from build123d import *

# Parameters (mm, degrees)
SKETCH_1_R               = 120
EXTRUDE_1_DEPTH          = 20
CUT_EXTRUDE_1_DEPTH      = 171.880074906
CUT_EXTRUDE_1_DEPTH_BACK = 171.880074906
SKETCH_2_R               = 15
CUT_EXTRUDE_2_DEPTH      = 15
PATTERN_CIRCULAR_1_COUNT = 3
SKETCH_5_R               = 1.5
CUT_EXTRUDE_3_DEPTH      = 171.880074906
PATTERN_CIRCULAR_2_COUNT = 3
CUT_EXTRUDE_4_DEPTH      = 171.880074906
PATTERN_CIRCULAR_3_COUNT = 3
SKETCH_7_R               = 20
CUT_EXTRUDE_5_DEPTH      = 171.880074906
SKETCH_8_R               = 1.5
CUT_EXTRUDE_6_DEPTH      = 171.880074906
PATTERN_CIRCULAR_4_COUNT = 3
SKETCH_12_W              = 5
SKETCH_12_H              = 25
EXTRUDE_3_DEPTH          = 10
EXTRUDE_4_DEPTH          = 4
PATTERN_CIRCULAR_5_COUNT = 3


with BuildPart() as part:
    # Sketch 1 → Extrude 1 (new body)
    with BuildSketch(Plane(origin=(0, 0, 0), x_dir=(1, 0, 0), z_dir=(0, 1, 0))):
        with Locations(Location((0, 0, 0), (0, 0, 270))):
            Circle(SKETCH_1_R)
    extrude(amount=EXTRUDE_1_DEPTH)

    # Sketch 2 → Cut-Extrude 1 (cut, two sides: drawn at the far end of the back side and taken through both)
    with BuildSketch(Plane(origin=(0, 20, 0), x_dir=(1, 0, 0), z_dir=(0, 1, 0)).offset(-CUT_EXTRUDE_1_DEPTH_BACK)):
        with Locations(Location((60, 0, 0), (0, 0, 270))):
            Circle(SKETCH_2_R)
        with Locations(Location((-30, -51.961524227, 0), (0, 0, 270))):
            Circle(SKETCH_2_R)
        with Locations(Location((-30, 51.961524227, 0), (0, 0, 270))):
            Circle(SKETCH_2_R)
    extrude(amount=CUT_EXTRUDE_1_DEPTH + CUT_EXTRUDE_1_DEPTH_BACK, mode=Mode.SUBTRACT)

    # Sketch 4 → Cut-Extrude 2 (cut)
    with BuildSketch(Plane.XZ):
        Polygon((7.009618943, 42.141016151), (32.990381057, 27.141016151), (82.990381057, 113.74355653), (57.009618943, 128.74355653), align=None)
    cut_extrude_2 = extrude(amount=-CUT_EXTRUDE_2_DEPTH, mode=Mode.SUBTRACT)

    # Pattern Circular 1: Cut-Extrude 2 ×3 about axis
    pattern_circular_1_axis = Axis((0, 0, 0), (0, 1, 0))
    for i in range(1, PATTERN_CIRCULAR_1_COUNT):
        add(cut_extrude_2.rotate(pattern_circular_1_axis, i * 360 / PATTERN_CIRCULAR_1_COUNT), mode=Mode.SUBTRACT)

    # Sketch 5 → Cut-Extrude 3 (cut, symmetric)
    with BuildSketch(Plane.XZ):
        with Locations(Location((-45, 0, 0), (0, 0, 270))):
            Circle(SKETCH_5_R)
        with Locations(Location((-75, 0, 0), (0, 0, 270))):
            Circle(SKETCH_5_R)
        with Locations(Location((-105, 0, 0), (0, 0, 270))):
            Circle(SKETCH_5_R)
    cut_extrude_3 = extrude(amount=CUT_EXTRUDE_3_DEPTH, both=True, mode=Mode.SUBTRACT)

    # Pattern Circular 2: Cut-Extrude 3 ×3 about axis
    pattern_circular_2_axis = Axis((0, 0, 0), (0, 1, 0))
    for i in range(1, PATTERN_CIRCULAR_2_COUNT):
        add(cut_extrude_3.rotate(pattern_circular_2_axis, i * 360 / PATTERN_CIRCULAR_2_COUNT), mode=Mode.SUBTRACT)

    # Sketch 6 → Cut-Extrude 4 (cut, symmetric)
    with BuildSketch(Plane(origin=(0, 20, 0), x_dir=(1, 0, 0), z_dir=(0, 1, 0))):
        with BuildLine():
            Line((41, 20), (41, -20))
            Line((41, -20), (50, -20))
            Line((50, -20), (50, -30))
            Line((50, -30), (70, -30))
            Line((70, -30), (70, -20))
            Line((70, -20), (96, -20))
            ThreePointArc((96, -20), (116, 0), (96, 20))
            Line((96, 20), (70, 20))
            Line((70, 20), (70, 30))
            Line((70, 30), (50, 30))
            Line((50, 30), (50, 20))
            Line((50, 20), (41, 20))
        make_face()
    cut_extrude_4 = extrude(amount=CUT_EXTRUDE_4_DEPTH, both=True, mode=Mode.SUBTRACT)

    # Pattern Circular 3: Cut-Extrude 4 ×3 about axis
    pattern_circular_3_axis = Axis((0, 0, 0), (0, 1, 0))
    for i in range(1, PATTERN_CIRCULAR_3_COUNT):
        add(cut_extrude_4.rotate(pattern_circular_3_axis, i * 360 / PATTERN_CIRCULAR_3_COUNT), mode=Mode.SUBTRACT)

    # Sketch 7 → Cut-Extrude 5 (cut, through all)
    with BuildSketch(Plane(origin=(0, 20, 0), x_dir=(1, 0, 0), z_dir=(0, 1, 0))):
        with Locations(Location((0, 0, 0), (0, 0, 270))):
            Circle(SKETCH_7_R)
    extrude(amount=-CUT_EXTRUDE_5_DEPTH, mode=Mode.SUBTRACT)

    # Sketch 8 → Cut-Extrude 6 (cut, symmetric)
    with BuildSketch(Plane(origin=(0, 20, 0), x_dir=(1, 0, 0), z_dir=(0, 1, 0))):
        with Locations(Location((-105, 27.5, 0), (0, 0, 270))):
            Circle(SKETCH_8_R)
        with Locations(Location((-105, -27.5, 0), (0, 0, 270))):
            Circle(SKETCH_8_R)
    cut_extrude_6 = extrude(amount=CUT_EXTRUDE_6_DEPTH, both=True, mode=Mode.SUBTRACT)

    # Pattern Circular 4: Cut-Extrude 6 ×3 about axis
    pattern_circular_4_axis = Axis((0, 0, 0), (0, 1, 0))
    for i in range(1, PATTERN_CIRCULAR_4_COUNT):
        add(cut_extrude_6.rotate(pattern_circular_4_axis, i * 360 / PATTERN_CIRCULAR_4_COUNT), mode=Mode.SUBTRACT)

    # Sketch 12 → Extrude 3 (add)
    with BuildSketch(Plane(origin=(0, 20, 0), x_dir=(1, 0, 0), z_dir=(0, 1, 0))):
        with Locations((-61.5, 0.5)):
            Rectangle(SKETCH_12_W, SKETCH_12_H)
    extrude_3 = extrude(amount=EXTRUDE_3_DEPTH)

    # Sketch 13 → Extrude 4 (add)
    with BuildSketch(Plane(origin=(0, 30, 0), x_dir=(1, 0, 0), z_dir=(0, 1, 0))):
        Polygon((-69, 8), (-59, 8), (-59, 13), (-64, 18), (-69, 18), align=None)
        Polygon((-59, -13), (-59, -8), (-69, -8), (-69, -18), (-64, -18), align=None)
    extrude_4 = extrude(amount=EXTRUDE_4_DEPTH)

    # Pattern Circular 5: Extrude 3, Extrude 4 ×3 about axis
    pattern_circular_5_axis = Axis((0, 0, 0), (0, 1, 0))
    add([extrude_3.rotate(pattern_circular_5_axis, i * 360 / PATTERN_CIRCULAR_5_COUNT) for i in range(1, PATTERN_CIRCULAR_5_COUNT)])
    add([extrude_4.rotate(pattern_circular_5_axis, i * 360 / PATTERN_CIRCULAR_5_COUNT) for i in range(1, PATTERN_CIRCULAR_5_COUNT)])


solid = part.part
Geometry check sheet. Reference: the model listing, model coordinates, mm. A direction names the side the tool comes from. Round coordinates to 2 decimals unless told otherwise and drop trailing zeros. Order: outer loops, then holes, each group sorted by start corner. A loop starts at its lowest first (then second) coordinate and runs counter-clockwise, first axis right, second up. Notation, with made-up numbers: M -29,-32 L -21,-32 A21 ccw -21,-28 Z; hole C 15,-29.5 d5. An arc over 180 degrees is marked long. Answer in a Markdown table with one row per item. Add a question column.
Item 1: Set-up check for faces 4 (the face through (21, 30, 63)), 5 (the face through (29.34, 25.35, -51.19)), 6 (the face through (-5.46, 10.14, 49.46)), 7 (the face through (-79, 7, 15)), 8 (the face through (19.818, 7.395, 34.746)): record each of +Z, -Z, +X, -X, +Y, -Y from which the full face is reachable in a straight line by a thin tool's end or side.
Item 2: Sectioned sample at A-A, the plane x = -35. Enter the section's corners in (y, z), plus the area to 3 significant figures.
Item 3: Depth check by flat-ended pin: pin 1 Ø6 at (y, z) = (22, -19.5) entering from -X; pin 2 Ø4 at (y, z) = (16, 18) entering from -X; pin 3 Ø6 at (x, y) = (84.5, 14.5) entering from -Z. Enter the tip coordinate at first touch or a pass-through.
Item 4: Draft check along Z on faces 1 (the face through (31.7, 24.9, 55.6)), 2 (the face through (52.48, 7.4, 60.9)), 3 (the face through (-64, 34, 13)). Enter one of: released by +Z, released by -Z, zero draft, split by the parting line, or undercut.
Item 5: Material ranges on L1, parallel to X at y = 17.7, z = 0; L2, parallel to X at y = 14, z = 0; L3, parallel to Z at x = -20.5, y = 17.5, recorded low to high. Write a range as [from, to].
Filled in:
| question | item | result |
|---|---|---|
| 1 | face 4 | +Z |
| 1 | face 5 | -X, +Y |
| 1 | face 6 | +Y, -Y |
| 1 | face 7 | -X, -Y |
| 1 | face 8 | -Y |
| 2 | outline | M 0,-114.78 L 20,-114.78 L 20,-98.34 L 0,-98.34 Z; M 0,-27.14 L 20,-27.14 L 20,27.14 L 0,27.14 Z; M 0,98.34 L 20,98.34 L 20,114.78 L 0,114.78 Z |
| 2 | area | 1,740 mm² |
| 3 | pin 1 | stops at x = -118.75 |
| 3 | pin 2 | stops at x = -118.93 |
| 3 | pin 3 | stops at z = -88.08 |
| 4 | face 1 | released by +Z |
| 4 | face 2 | undercut |
| 4 | face 3 | zero draft |
| 5 | L1 | x = [-120, -106.5], [-103.5, -76.5], [-73.5, -46.5], [-43.5, -20], [20, 41], [116, 120] |
| 5 | L2 | x = [-40, -20], [20, 41], [116, 120] |
| 5 | L3 | z = [-118.24, -75.51], [-35.51, 35.51], [75.51, 118.24] |
